from build123d import *

# Parameters (mm, degrees)
SKETCH1_W           = 76.2
SKETCH1_H           = 88.9
BOSS_EXTRUDE1_DEPTH = 3.175
SKETCH2_R           = 3.175
SKETCH2_R_2         = 10.99185
CUT_EXTRUDE1_DEPTH  = 7.35
CUT_EXTRUDE2_REACH  = 8.35
SKETCH5_R           = 3.175
SKETCH5_W           = 25.4
SKETCH5_H           = 25.4


with BuildPart() as part:
    # Sketch1 → Boss-Extrude1 (new body, symmetric)
    with BuildSketch(Plane.XY):
        with Locations((38.1, 44.45)):
            Rectangle(SKETCH1_W, SKETCH1_H)
    extrude(amount=BOSS_EXTRUDE1_DEPTH, both=True)

    # Sketch2 → Cut-Extrude1 (cut, through all)
    with BuildSketch(Plane.XY.offset(3.175)):
        with Locations((12.7, 76.2)):
            Circle(SKETCH2_R)
        with Locations((63.5, 76.2)):
            Circle(SKETCH2_R)
        with Locations((63.5, 12.7)):
            Circle(SKETCH2_R)
        with Locations((12.7, 12.7)):
            Circle(SKETCH2_R)
        with Locations((38.1, 36.83)):
            Circle(SKETCH2_R_2)
        with Locations((12.7, 57.15)):
            Circle(SKETCH2_R)
        with Locations((63.5, 57.15)):
            Circle(SKETCH2_R)
    extrude(amount=-CUT_EXTRUDE1_DEPTH, mode=Mode.SUBTRACT)

    # Sketch5 → Cut-Extrude2 (cut, up to next)
    with BuildSketch(Plane.XY.offset(3.175), mode=Mode.PRIVATE) as cut_extrude2_sk1:
        with Locations((38.1, 76.2)):
            Circle(SKETCH5_R)
    cut_extrude2_tool1 = extrude(cut_extrude2_sk1.sketch, amount=-CUT_EXTRUDE2_REACH, mode=Mode.PRIVATE) & part.part
    add(cut_extrude2_tool1.solids().sort_by_distance((38.1, 76.2, 3.175))[0], mode=Mode.SUBTRACT)
    # Sketch5 → Cut-Extrude2 (cut, up to next)
    with BuildSketch(Plane.XY.offset(3.175), mode=Mode.PRIVATE) as cut_extrude2_sk2:
        with Locations((63.5, 76.2)):
            Rectangle(SKETCH5_W, SKETCH5_H)
    cut_extrude2_tool2 = extrude(cut_extrude2_sk2.sketch, amount=-CUT_EXTRUDE2_REACH, mode=Mode.PRIVATE) & part.part
    add(cut_extrude2_tool2.solids().sort_by_distance((63.5, 76.2, 3.175))[0], mode=Mode.SUBTRACT)
    # Sketch5 → Cut-Extrude2 (cut, up to next)
    with BuildSketch(Plane.XY.offset(3.175), mode=Mode.PRIVATE) as cut_extrude2_sk3:
        with Locations((12.7, 76.2)):
            Rectangle(SKETCH5_W, SKETCH5_H)
    cut_extrude2_tool3 = extrude(cut_extrude2_sk3.sketch, amount=-CUT_EXTRUDE2_REACH, mode=Mode.PRIVATE) & part.part
    add(cut_extrude2_tool3.solids().sort_by_distance((12.7, 76.2, 3.175))[0], mode=Mode.SUBTRACT)


solid = part.part
Input: part model. Units: mm. Frame: model coordinates. A direction names the side the tool comes from. Give positions to 0.01 mm unless a question says otherwise; leave off trailing zeros. Loops run counter-clockwise (first coordinate to the right, second up) from the corner with the lowest first, then second, coordinate; pieces in that order, holes last. Notation, with made-up numbers: M 28,38.5 L 80,38.5 A18 cw 80,48.5 Z; hole C 2,-39 d2. An arc over 180 degrees is marked long. Use one line per item in the form item = value.
1. Section query A-A, the plane x = 38.1. Return the cut outline in (y, z) (3 decimals).
Numbers:
outline = M 0,-3.175 L 25.838,-3.175 L 25.838,3.175 L 0,3.175 Z; M 47.822,-3.175 L 73.025,-3.175 L 73.025,3.175 L 47.822,3.175 Z; M 79.375,-3.175 L 88.9,-3.175 L 88.9,3.175 L 79.375,3.175 Z
2. First-contact query: pin 1 (1.9 mm diameter, centred on y = 82, z = 0.5, fed in from +X); pin 2 (8.5 mm diameter, centred on x = 63.5, y = 57.15, fed in from -Z) (3 decimals); pin 3 (4 mm diameter, centred on x = 12.7, y = 57.15, fed in from -Z); pin 4 (1.9 mm diameter, centred on x = 59.5, z = 0.5, fed in from +Y). Flat tips, straight axial feed; report the tip coordinate or a pass-through.
Numbers:
pin_1 = 50.8
pin_2 = -3.175
pin_3 = through
pin_4 = 63.5
3. Pull-direction query (Y, two-part tool) for faces 1 (the face through (30, 44.26, 0.04)), 2 (the face through (76.2, 31, 0)), 3 (the face through (38, 0, 0)), 4 (the face through (13, 63.5, 0)); classes: released by +Y, released by -Y, zero draft, split by the parting line, or undercut.
Numbers:
face_1 = undercut
face_2 = zero draft
face_3 = released by -Y
face_4 = released by +Y
4. Line query: L1, parallel to Y at x = 12.7, z = 0 (3 decimals); L2, parallel to Y at x = 38.1, z = 0 (3 decimals); L3, parallel to X at y = 12.5, z = -2.25. Output: solid intervals per line, ascending.
Numbers:
L1 = 0 to 9.525, 15.875 to 53.975, 60.325 to 63.5
L2 = 0 to 25.838, 47.822 to 73.025, 79.375 to 88.9
L3 = 0 to 9.53, 15.87 to 60.33, 66.67 to 76.2
5. Section query B-B, the plane y = 36.83. Return the cut outline in (x, z) (3 decimals).
Numbers:
outline = M 0,-3.175 L 27.108,-3.175 L 27.108,3.175 L 0,3.175 Z; M 49.092,-3.175 L 76.2,-3.175 L 76.2,3.175 L 49.092,3.175 Z
6. Section query C-C, the plane y = 12.7. Return the cut outline in (x, z) (3 decimals), and give its area (3 significant figures).
Numbers:
outline = M 0,-3.175 L 9.525,-3.175 L 9.525,3.175 L 0,3.175 Z; M 15.875,-3.175 L 60.325,-3.175 L 60.325,3.175 L 15.875,3.175 Z; M 66.675,-3.175 L 76.2,-3.175 L 76.2,3.175 L 66.675,3.175 Z
area = 403 mm²
7. Reachability of faces 5 (the face through (25.4, 76, 0)), 6 (the face through (64.965, 54.333, 0.044)), 7 (the face through (50.8, 76, 0)) from +Z, -Z, +X, -X, +Y, -Y: full face, straight path, thin tool, end or side. Return the list, or none.
Numbers:
face_5 = +Z, -Z, -X, +Y
face_6 = +Z, -Z
face_7 = +Z, -Z, +X, +Y
8. Section query D-D, the plane z = 0.75. Return the cut outline in (x, y) (3 decimals), and give its area (3 significant figures).
Numbers:
outline = M 0,0 L 76.2,0 L 76.2,63.5 L 50.8,63.5 L 50.8,88.9 L 25.4,88.9 L 25.4,63.5 L 0,63.5 Z; hole C 12.7,12.7 d6.35; hole C 12.7,57.15 d6.35; hole C 38.1,36.83 d21.984; hole C 38.1,76.2 d6.35; hole C 63.5,12.7 d6.35; hole C 63.5,57.15 d6.35
area = 4,950 mm²
